The figure shows three views and two pictorial views of one solid part (mm, origin at its lowest corner). Answer the questions. A direction names the side the tool comes from. Coordinates: 2 decimals unless noted, no trailing zeros. Write each loop counter-clockwise with the first axis right and the second up, starting at its lowest first coordinate (ties: lowest second). Pieces come first, ordered by that corner, then holes. Notation, with made-up numbers: M 76,-5 L 119,-5 A22 ccw 119,18 Z; hole C 28.25,55 d7. An arc over 180 degrees is marked long. Use CSV: the item, a comma, the result in double quotes.
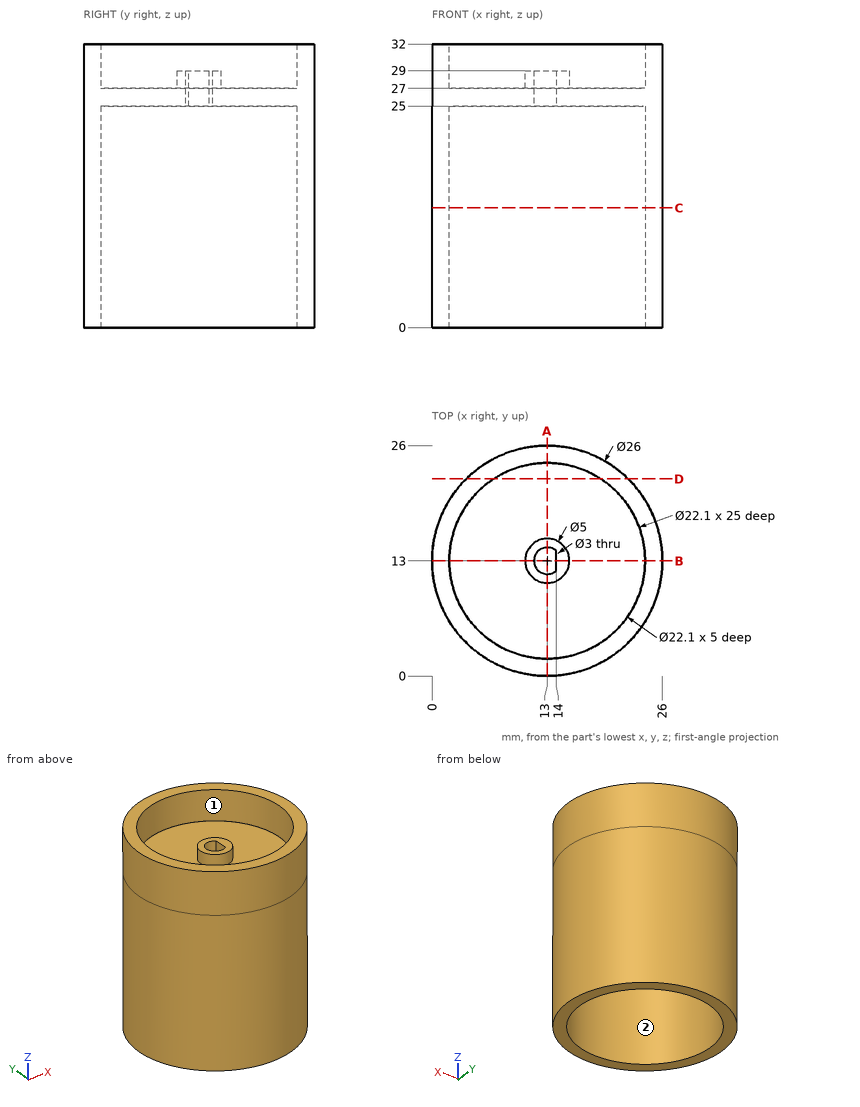
Item 1: The part is cut by section B-B (y = 13). Write down the section's boundary in (x, z).
Answer:
outline,"M 0,0 L 1.95,0 L 1.95,25 L 11.5,25 L 11.5,29 L 10.5,29 L 10.5,27 L 1.95,27 L 1.95,32 L 0,32 Z; M 14,25 L 24.05,25 L 24.05,0 L 26,0 L 26,32 L 24.05,32 L 24.05,27 L 15.5,27 L 15.5,29 L 14,29 Z"
Item 2: The part is cut by section C-C (z = 13.5). Write down the section's boundary in (x, y).
Answer:
outline,"C 13,13 d26; hole C 13,13 d22.1"
Item 3: The part is cut by section A-A (x = 13). Write down the section's boundary in (y, z), then the cut area to 3 significant figures.
Answer:
outline,"M 0,0 L 1.95,0 L 1.95,25 L 11.5,25 L 11.5,29 L 10.5,29 L 10.5,27 L 1.95,27 L 1.95,32 L 0,32 Z; M 14.5,25 L 24.05,25 L 24.05,0 L 26,0 L 26,32 L 24.05,32 L 24.05,27 L 15.5,27 L 15.5,29 L 14.5,29 Z"
area,"167 mm2"
Item 4: Consider probe 1 along Y at (x, z) = (13, 26.9); probe 2 along Y at (x, z) = (19, 20.5); probe 3 along X at (y, z) = (10, 5). Determine where each line is inside the solid, lowest interval first.
Answer:
probe 1,"y = 0 to 11.5, 14.5 to 26"
probe 2,"y = 1.47 to 3.72, 22.28 to 24.53"
probe 3,"x = 0.35 to 2.37, 23.63 to 25.65"
Item 5: Given pin 1 (1.5 mm diameter, centred on x = 16.5, y = 8.5, fed in from -Z); pin 2 (1.5 mm diameter, centred on y = 14, z = 28.5, fed in from -X); pin 3 (2 mm diameter, centred on y = 22, z = 26.5, fed in from +X); pin 4 (1.8 mm diameter, centred on x = 13, y = 13, fed in from +Z), each flat-ended and moving along its own axis, determine where each tip first touches the part or whether it passes through.
Answer:
pin 1,"stops at z = 25"
pin 2,"stops at x = 0"
pin 3,"stops at x = 23.25"
pin 4,"passes through"
Item 6: The part is cut by section D-D (y = 22.25). Write down the section's boundary in (x, z), then the cut area to 3 significant figures.
Answer:
outline,"M 3.87,0 L 6.96,0 L 6.96,25 L 19.04,25 L 19.04,0 L 22.13,0 L 22.13,32 L 19.04,32 L 19.04,27 L 6.96,27 L 6.96,32 L 3.87,32 Z"
area,"222 mm2"
Item 7: A tool of negligible diameter and unlimited length cuts with its end or side. For the marked faces 1 and 2, from which of +Z, -Z, +X, -X, +Y, -Y can it reach the whole face along a straight path? Write none if from no direction.
Answer:
face 1,"+Z"
face 2,"-Z"
